from build123d import *

# Parameters (mm, degrees)
SKETCH1_W           = 22.125
SKETCH1_H           = 22.125
SKETCH1_W_2         = 19.15
SKETCH1_H_2         = 19.15
BOSS_EXTRUDE1_DEPTH = 12.7
CUT_EXTRUDE1_DEPTH  = 12.7


with BuildPart() as part:
    # Sketch1 → Boss-Extrude1 (new body, symmetric)
    with BuildSketch(Plane.XY):
        with Locations((-2.278232981, -0.982857981)):
            Rectangle(SKETCH1_W, SKETCH1_H)
        with Locations((-1.182857981, -0.982857981)):
            Rectangle(SKETCH1_W_2, SKETCH1_H_2, mode=Mode.SUBTRACT)
    extrude(amount=BOSS_EXTRUDE1_DEPTH, both=True)

    # Sketch2 → Cut-Extrude1 (cut)
    with BuildSketch(Plane.ZY.offset(13.340732981)):
        with BuildLine():
            Line((-3.175, 1.557142019), (12.7, 1.557142019))
            Line((12.7, 1.557142019), (12.7, -3.522857981))
            Line((12.7, -3.522857981), (-3.175, -3.522857981))
            ThreePointArc((-3.175, -3.522857981), (-5.715, -0.982857981), (-3.175, 1.557142019))
        make_face()
    extrude(amount=-CUT_EXTRUDE1_DEPTH, mode=Mode.SUBTRACT)


solid = part.part
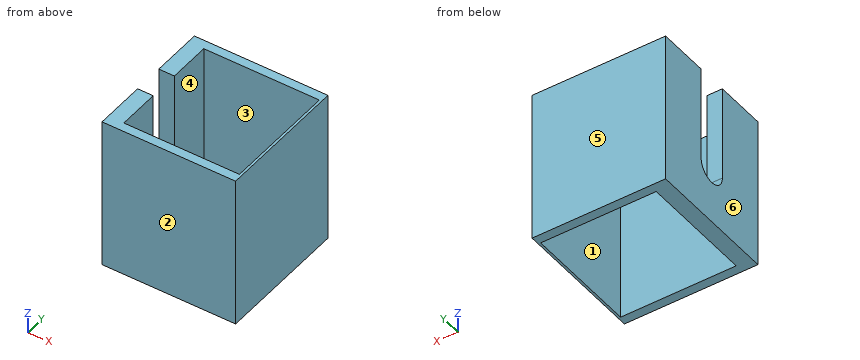
Could you check a few things on this model? Use its own coordinates, in mm. Face numbers are marked on the shaded views. A direction names the side the tool comes from. Give positions to 0.01 mm unless a question says otherwise; leave off trailing zeros. Order: outer loops, then holes, each group sorted by start corner. A loop starts at its lowest first (then second) coordinate and runs counter-clockwise, first axis right, second up.
1. Thinking about a two-plate mould opening in X: for the marked faces 3, 4, 5 and 6, which applies, +X half, -X half, draft (parallel to the pull), parting line (faces both ways), or undercut?
Answers below:
face 3: undercut
face 4: undercut
face 5: draft
face 6: -X half
2. I need wall thicknesses on L1, parallel to Y at x = -6, z = 1.5; L2, parallel to X at y = -2.75, z = -5.25; L3, parallel to Y at x = -11.25, z = 11.75. Which ranges of each line are inside material? Lowest first, please.
Answers below:
L1: y = -12.05 to -10.56, 8.59 to 10.08
L2: x = -13.34 to -10.76, 8.39 to 8.78
L3: y = -12.05 to -3.52, 1.56 to 10.08
3. Which directions (+Z, -Z, +X, -X, +Y, -Y) give clear straight access to the entire face, cutting with the end or side of a thin tool? Please do the marked faces 1 and 2.
Answers below:
face 1: +Z, -Z
face 2: +Z, -Z, +X, -X, -Y
4. Suppose I cut it at B-B (x = 1.75). Write out the boundary of the cut face in (y, z), plus the area to 3 significant figures.
Answers below:
outline: (-12.05, -12.7) - (-10.56, -12.7) - (-10.56, 12.7) - (-12.05, 12.7) - close; (8.59, -12.7) - (10.08, -12.7) - (10.08, 12.7) - (8.59, 12.7) - close
area: 75.6 mm2
5. Suppose I cut it at A-A (y = 4.5). Write out the boundary of the cut face in (x, z), plus the area to 3 significant figures.
Answers below:
outline: (-13.34, -12.7) - (-10.76, -12.7) - (-10.76, 12.7) - (-13.34, 12.7) - close; (8.39, -12.7) - (8.78, -12.7) - (8.78, 12.7) - (8.39, 12.7) - close
area: 75.6 mm2
6. For pin 1 (4 mm diameter, centred on x = 3.5, y = 5.5, fed in from -Z), with a flat end and sliding along its axis, tell me the tip position at first contact or that it passes through.
Answers below:
pin 1: passes through
7. Suppose I cut it at C-C (z = -9.25). Write out the boundary of the cut face in (x, y).
Answers below:
outline: (-13.34, -12.05) - (8.78, -12.05) - (8.78, 10.08) - (-13.34, 10.08) - close; hole (-10.76, -10.56) - (8.39, -10.56) - (8.39, 8.59) - (-10.76, 8.59) - close
8. Suppose I cut it at D-D (z = 6). Write out the boundary of the cut face in (x, y), plus the area to 3 significant figures.
Answers below:
outline: (-13.34, -12.05) - (8.78, -12.05) - (8.78, 10.08) - (-13.34, 10.08) - (-13.34, 1.56) - (-10.76, 1.56) - (-10.76, 8.59) - (8.39, 8.59) - (8.39, -10.56) - (-10.76, -10.56) - (-10.76, -3.52) - (-13.34, -3.52) - close
area: 110 mm2
